from build123d import *

# Parameters (mm, degrees)
BOX_W              = 13.4
BOX_H              = 13.4
BOX_DEPTH          = 14
SKETCH001_R        = 24
POCKET_DEPTH       = 6
POLARPATTERN_COUNT = 5


with BuildPart() as cube:
    # Box → Box (new body)
    with BuildSketch(Plane(origin=(-6.7, -6.7, 10), x_dir=(1, 0, 0), z_dir=(0, 0, 1))):
        with Locations((6.7, 6.7)):
            Rectangle(BOX_W, BOX_H)
    extrude(amount=BOX_DEPTH)


with BuildPart() as body:
    # Sketch → Revolve (revolve)
    with BuildSketch(Plane.XZ):
        with BuildLine():
            Line((91.081299, 18.37), (105, 18.37))
            Line((105, 18.37), (97.032315, 21.27))
            Line((97.032315, 21.27), (97.032315, 23.77))
            Line((97.032315, 23.77), (105, 26.67))
            Line((105, 26.67), (4.86, 26.67))
            Line((4.86, 26.67), (4.86, 10.010664))
            Line((4.86, 10.010664), (11.05, 10.010664))
            Line((11.05, 10.010664), (11.05, 18.37))
            add(Edge.make_bspline(
                [(91.081299, 18.37), (58.452015, 25.146616), (31.574902, 25.049244), (11.05, 18.37)],
                knots=[0, 0, 0, 0, 1, 1, 1, 1], degree=3))
        make_face()
    revolve(axis=Axis((0, 0, 0), (0, 0, 1)))

    # Cut: cut Cube
    add(cube.part, mode=Mode.SUBTRACT)

    # Sketch001 (on Face12 of BaseFeature) → Pocket (cut)
    with BuildSketch(Plane.XY.offset(26.67)):
        with Locations((-35.831062, 36.219181)):
            Circle(SKETCH001_R)
    pocket = extrude(amount=-POCKET_DEPTH, mode=Mode.SUBTRACT)

    # PolarPattern: Pocket ×5 about axis
    polarpattern_axis = Axis((0, 0, 26.67), (0, 0, 1))
    for i in range(1, POLARPATTERN_COUNT):
        add(pocket.rotate(polarpattern_axis, i * 360 / POLARPATTERN_COUNT), mode=Mode.SUBTRACT)


solid = body.part
Verification items for the finished model (mm, model axes). A direction names the side the tool comes from. Give positions to 0.01 mm unless a question says otherwise; leave off trailing zeros. Loops run counter-clockwise (first coordinate to the right, second up) from the corner with the lowest first, then second, coordinate; pieces in that order, holes last. Notation, with made-up numbers: (44.25, -36) - (61.25, -36) arc R25 ccw to (61.25, -14) - close; hole circle Ø11 at (12.25, 5). An arc over 180 degrees is marked (long way). Write item = value, one per line. Start each with the question number.
Q1. Cross-section at A-A, the plane z = 15.75. Enter the section's corners in (x, y), and give its area (3 significant figures).
Q2. Thickness scan on line 1 (X direction, y = 50, z = 23.5); line 2 (Z direction, x = 48.5, y = 83.5); line 3 (X direction, y = -70, z = 23.5). Record the ranges inside material, lowest first.
Q3. Tool access check on faces 5 (the face through (-1, -22, 26.67)), 6 (the face through (0, -6.7, 17)), 7 (the face through (-21.14, -95.21, 23.95)). Record the directions out of +Z, -Z, +X, -X, +Y, -Y that give a thin tool (end or side, any length) a straight path to the whole face; none if there is none.
Q4. Mould release check, pull along Y, two halves, no side actions. Record for faces 1 (the face through (-66.41, -34.7, 24.59)), 2 (the face through (-21.12, -95.1, 21.13)), 3 (the face through (-53.52, 52.44, 24.59)), 4 (the face through (0, -7, 10.011)): released by +Y, released by -Y, zero draft, split by the parting line, or undercut.
Q5. Cross-section at B-B, the plane y = 40. State how many separate pieces and enclosed holes the cut face has, and give its area (3 significant figures).
Q6. Depth check by flat-ended pin: P1, Ø4, axis at y = 2, z = 16, coming from the -X side; P2, Ø4, axis at y = -84, z = 16, coming from the -X side; P3, Ø4, axis at x = -1, y = -3, coming from the -Z side; P4, Ø4, axis at x = -1.5, z = 13.5, coming from the +Y side. Enter the tip coordinate at first touch or a pass-through.
Answer key:
q1.outline = circle Ø22.1 at (0, 0); hole (-6.7, -6.7) - (6.7, -6.7) - (6.7, 6.7) - (-6.7, 6.7) - close
q1.area = 204 mm^2
q2.line_1 = -83.16 to -55.48, -16.18 to -0.16, 46.9 to 83.16
q2.line_2 = 18.37 to 26.67
q2.line_3 = -67.2 to -6.1, 21.5 to 67.2
q3.face_5 = +Z, +X, -X, +Y, -Y
q3.face_6 = -Z
q3.face_7 = none
q4.face_1 = undercut
q4.face_2 = split by the parting line
q4.face_3 = undercut
q4.face_4 = zero draft
q5.separate_pieces = 3
q5.enclosed_holes = 0
q5.area = 546 mm^2
q6.P1 = -11.05
q6.P2 = through
q6.P3 = 24
q6.P4 = 11.05
